```python
from build123d import *

# Parameters (mm, degrees)
F0_R     = 2.7
F0_R_2   = 1.45
F1_DEPTH = 3
F2_DEPTH = 28
F4_DEPTH = 2
F5_R     = 0.2


with BuildPart() as f1:
    # F0 (on Top) → F1 (new body)
    with BuildSketch(Plane.XY):
        with Locations((-51.408798, -20.234108)):
            Circle(F0_R)
        with Locations((-51.408798, -20.234108)):
            Circle(F0_R_2, mode=Mode.SUBTRACT)
        with Locations((-51.408798, -20.234108)):
            Circle(F0_R_2)
    extrude(amount=F1_DEPTH)

    # F0 (on Top) → F2 (join)
    with BuildSketch(Plane.XY):
        with Locations((-51.408798, -20.234108)):
            Circle(F0_R_2)
    extrude(amount=F2_DEPTH)

    # F3 (on face) → F4 (cut)
    with BuildSketch(Plane(origin=(0, 0, 0), x_dir=(1, 0, 0), z_dir=(0, 0, -1))):
        Polygon((-52.130485, 18.984108), (-50.68711, 18.984108), (-49.965422, 20.234108), (-50.68711, 21.484108), (-52.130485, 21.484108), (-52.852173, 20.234108), align=None)
    extrude(amount=-F4_DEPTH, mode=Mode.SUBTRACT)

    # F5
    f5_edges = [f1.edges().sort_by_distance(p)[0] for p in [
        (-54.108798, -20.234108, 0),
        (-51.408798, -18.984108, 2),
        (-50.326266, -19.609108, 2),
        (-50.326266, -20.859108, 2),
        (-51.408798, -21.484108, 2),
        (-52.491329, -20.859108, 2),
        (-52.491329, -19.609108, 2),
        (-52.491329, -19.609108, 0),
        (-52.491329, -20.859108, 0),
        (-51.408798, -21.484108, 0),
        (-50.326266, -20.859108, 0),
        (-50.326266, -19.609108, 0),
        (-51.408798, -18.984108, 0),
    ]]
    fillet(f5_edges, radius=F5_R)


solid = f1.part
```
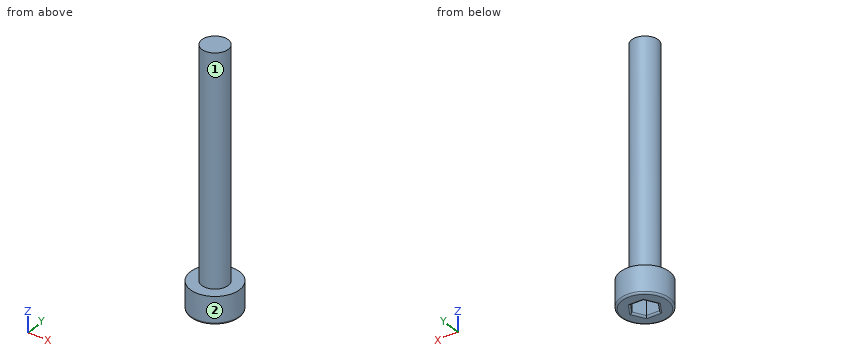
Check sheet for the modelled part. Datum: model origin and axes. Units: mm. Face numbers are marked on the shaded views. A direction names the side the tool comes from. Round coordinates to 2 decimals unless told otherwise and drop trailing zeros. Order: outer loops, then holes, each group sorted by start corner. A loop starts at its lowest first (then second) coordinate and runs counter-clockwise, first axis right, second up. Notation, with made-up numbers: M 36.5,-3 L 65.5,-3 A23 ccw 65.5,34 Z; hole C 50.5,62 d4. An arc over 180 degrees is marked long. Answer in a Markdown table with one row per item.
(1) Gauge pin test, flat ends, axial feed: pin 1 (2 mm diameter, centred on y = -18, z = 12.5, fed in from -X); pin 2 (1.7 mm diameter, centred on x = -52, y = -20.5, fed in from -Z); pin 3 (2 mm diameter, centred on x = -52, z = 23.5, fed in from -Y). Record the tip position at first contact, or that the pin passes through.
Findings:
| item | result |
|---|---|
| pin 1 | stops at x = -52.17 |
| pin 2 | stops at z = 0 |
| pin 3 | stops at y = -21.68 |
(2) Set-up check for the marked faces 1 and 2: record each of +Z, -Z, +X, -X, +Y, -Y from which the full face is reachable in a straight line by a thin tool's end or side.
Findings:
| item | result |
|---|---|
| face 1 | +Z |
| face 2 | +Z, -Z |
(3) Material ranges on line 1 along Z through (x, y) = (-53.6, -20.6); line 2 along Y through (x, z) = (-51.5, 18.75); line 3 along Z through (x, y) = (-51.95, -19.4), recorded low to high. Write a range as from..to.
Findings:
| item | result |
|---|---|
| line 1 | z = 0..3 |
| line 2 | y = -21.68..-18.79 |
| line 3 | z = 2..28 |
(4) Section check A-A on z = 9. Record the boundary of the cut face in (x, y), plus the area to 3 significant figures.
Findings:
| item | result |
|---|---|
| outline | C -51.41,-20.23 d2.9 |
| area | 6.61 mm^2 |
